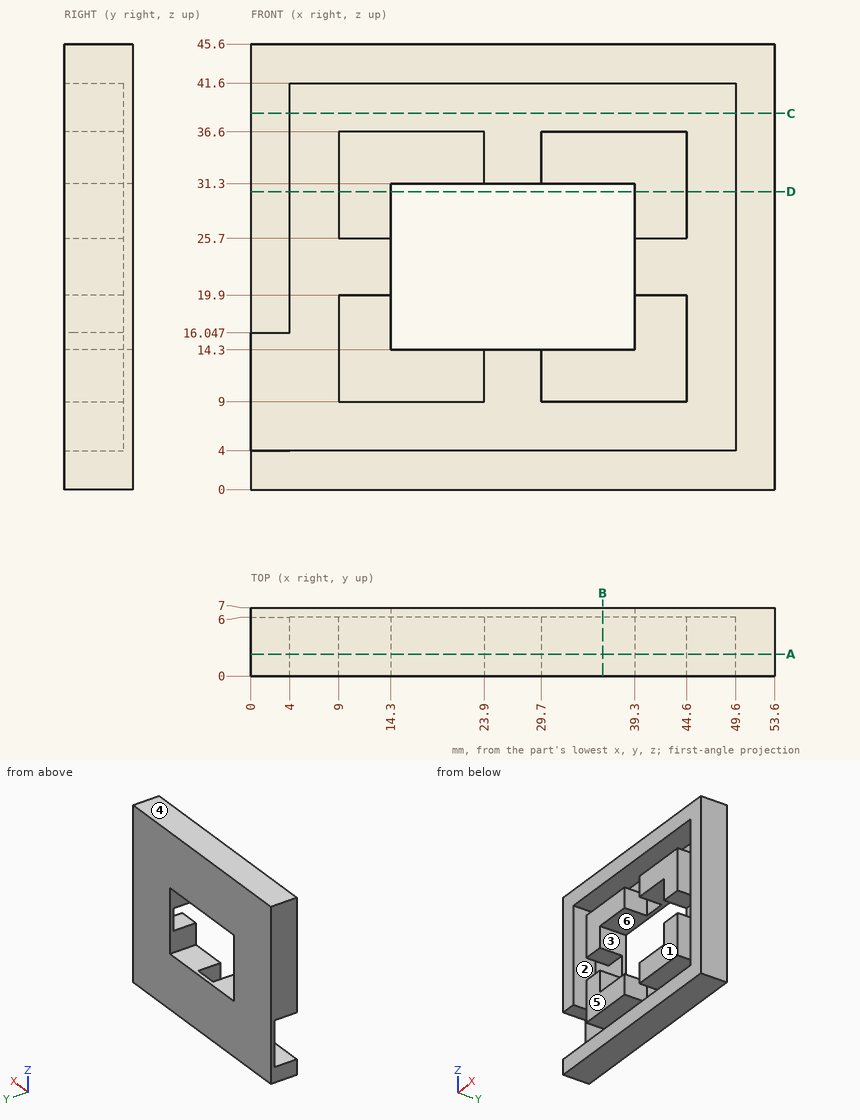
Input: dimensioned drawing with shaded views. Units: mm. Origin: part minimum x, y, z. A direction names the side the tool comes from. Round coordinates to 2 decimals unless told otherwise and drop trailing zeros. Order: outer loops, then holes, each group sorted by start corner. A loop starts at its lowest first (then second) coordinate and runs counter-clockwise, first axis right, second up. Notation, with made-up numbers: (-35.75, 86.25) -> (-0.75, 86.25) arc R22 cw to (-0.75, 116.25) -> close; hole circle Ø5 at (-26, -27.5). An arc over 180 degrees is marked (long way). One line per item, written item: value. Start each with the question number.
Q1. Section query A-A (y = 2.25). Give the number of separate pieces and of enclosed holes in the cut face, plus the area to 3 significant figures.
Q2. Access query for the marked faces 1, 2 and 3. Directions: +Z, -Z, +X, -X, +Y, -Y. A direction counts if a zero-diameter tool reaches every point of the face in a straight line with its end or side. Return the directions, or none.
Q3. Section query D-D (z = 30.5). Return the cut outline in (x, y).
Q4. Pin query (flat end, axial travel): pin 1 (3 mm diameter, centred on x = 16.5, y = 3.5, fed in from -Z). Return the tip coordinate at first contact, or that it passes through.
Q5. Section query B-B (x = 36). Return the cut outline in (y, z), plus the area to 3 significant figures.
Q6. Material intervals for probe 1 along Z at (x, y) = (13, 1.25); probe 2 along X at (y, z) = (4.5, 16.5); probe 3 along Z at (x, y) = (34, 2), sorted ascending.
Q7. Draft query along Z for the marked faces 4, 5 and 6. Return one class per face: pulls with the +Z half, pulls with the -Z half, needs draft (parallel to the pull), parting line crosses it, or undercut.
Q8. Section query C-C (z = 38.5). Return the cut outline in (x, y).
Findings below:
1. separate pieces: 5
1. enclosed holes: 0
1. area: 1,120 mm²
2. face 1: +Z, -Z, +X, -X, -Y
2. face 2: -Y
2. face 3: +Y, -Y
3. outline: (0, 0) -> (4, 0) -> (4, 6) -> (9, 6) -> (9, 0) -> (14.3, 0) -> (14.3, 7) -> (0, 7) -> close; (39.3, 0) -> (44.6, 0) -> (44.6, 6) -> (49.6, 6) -> (49.6, 0) -> (53.6, 0) -> (53.6, 7) -> (39.3, 7) -> close
4. pin 1: z = 0
5. outline: (0, 0) -> (7, 0) -> (7, 14.3) -> (0, 14.3) -> (0, 9) -> (6, 9) -> (6, 4) -> (0, 4) -> close; (0, 31.3) -> (7, 31.3) -> (7, 45.6) -> (0, 45.6) -> (0, 41.6) -> (6, 41.6) -> (6, 36.6) -> (0, 36.6) -> close
5. area: 140 mm²
6. probe 1: 0 to 4, 9 to 19.9, 25.7 to 36.6, 41.6 to 45.6
6. probe 2: 0 to 4, 9 to 14.3, 39.3 to 44.6, 49.6 to 53.6
6. probe 3: 0 to 4, 9 to 14.3, 31.3 to 36.6, 41.6 to 45.6
7. face 4: pulls with the +Z half
7. face 5: needs draft
7. face 6: undercut
8. outline: (0, 0) -> (4, 0) -> (4, 6) -> (49.6, 6) -> (49.6, 0) -> (53.6, 0) -> (53.6, 7) -> (0, 7) -> close
